from build123d import *

# Parameters (mm, degrees)
SKETCH1_R               = 51.562
SKETCH1_R_2             = 50.8
BOSS_EXTRUDE1_DEPTH     = 300
CUT_EXTRUDE1_DEPTH      = 309.73496674
CUT_EXTRUDE1_DEPTH_BACK = 309.73496674
SKETCH3_R               = 6.35
SKETCH4_R               = 3.048
SKETCH4_R_2             = 2.54
CUT_EXTRUDE2_DEPTH      = 309.734966871
CIRPATTERN1_COUNT       = 2
CIRPATTERN1_ANGLE       = 90


with BuildPart() as part:
    # Sketch1 → Boss-Extrude1 (new, symmetric)
    with BuildSketch(Plane(origin=(0, 0, 0), x_dir=(0, 0, -1), z_dir=(1, 0, 0))):
        Circle(SKETCH1_R)
        Circle(SKETCH1_R_2, mode=Mode.SUBTRACT)
    extrude(amount=BOSS_EXTRUDE1_DEPTH, both=True)

    # Sketch3 → Cut-Extrude1 (cut, two sides: drawn at the far end of the back side and taken through both)
    with BuildSketch(Plane.XY.offset(-CUT_EXTRUDE1_DEPTH_BACK)):
        with Locations((170.180000052, -8.89)):
            Circle(SKETCH3_R)
    extrude(amount=CUT_EXTRUDE1_DEPTH + CUT_EXTRUDE1_DEPTH_BACK, mode=Mode.SUBTRACT)

    # Sketch4 → Cut-Extrude2 (cut, symmetric)
    with BuildSketch(Plane.XY):
        with Locations((-287.3, 0)):
            Circle(SKETCH4_R)
        with Locations((289.586, 0)):
            Circle(SKETCH4_R_2)
    cut_extrude2 = extrude(amount=CUT_EXTRUDE2_DEPTH, both=True, mode=Mode.SUBTRACT)

    # CirPattern1: Cut-Extrude2 ×2 about axis
    cirpattern1_axis = Axis((300, 0, 0), (-1, 0, 0))
    for i in range(1, CIRPATTERN1_COUNT):
        add(cut_extrude2.rotate(cirpattern1_axis, i * CIRPATTERN1_ANGLE / (CIRPATTERN1_COUNT - 1)), mode=Mode.SUBTRACT)


solid = part.part
Work out the finished part from the listing and answer in its coordinate system (mm). Give positions to 0.01 mm unless a question says otherwise; leave off trailing zeros. Loops run counter-clockwise (first coordinate to the right, second up) from the corner with the lowest first, then second, coordinate; pieces in that order, holes last. Notation, with made-up numbers: (45.25, 62) - (80.25, 62) arc R21 cw to (80.25, 77) - close; hole circle Ø11 at (66.25, -31). An arc over 180 degrees is marked (long way). Answer in a Markdown table with one row per item. Add a question column.
Q1. The part is cut by section B-B (y = 33.5). Determine the outline of the cut face in (x, z).
Q2. Consider line 1 along X through (y, z) = (-51, 0); line 2 along Y through (x, z) = (4, 0); line 3 along Y through (x, z) = (167.5, -41). Determine where each line is inside the solid, lowest interval first.
Q3. Each of these flat-tipped pins is pushed along its axis until it touches: P1, Ø5, axis at x = 60, z = -21.5, coming from the -Y side; P2, Ø10, axis at x = -148, z = 13.5, coming from the -Y side; P3, Ø2, axis at x = 134, z = -16.5, coming from the -Y side. Where does it stop, or does it pass through?
Q4. Determine the mould class of faces 1 (the cylindrical face through (165.256, -12.9, -49.762)), 2 (the flat face through (-300, -38, -34)), 3 (the flat face through (300, -38, -34)) for opening direction X: released by +X, released by -X, zero draft, split by the parting line, or undercut.
Q5. The part is cut by section C-C (x = 245). Determine the outline of the cut face in (y, z), and give its area (3 significant figures).
Q6. The part is cut by section A-A (z = -31). Determine the outline of the cut face in (x, y).
Solution:
| question | item | result |
|---|---|---|
| 1 | outline | (-300, -39.2) - (300, -39.2) - (300, -38.19) - (-300, -38.19) - close; (-300, 38.19) - (300, 38.19) - (300, 39.2) - (-300, 39.2) - close |
| 2 | line 1 | x = -300 to -290.35, -284.25 to 287.05, 292.13 to 300 |
| 2 | line 2 | y = -51.56 to -50.8, 50.8 to 51.56 |
| 2 | line 3 | y = -31.27 to -29.99, 29.99 to 31.27 |
| 3 | P1 | stops at y = -47.93 |
| 3 | P2 | stops at y = -50.86 |
| 3 | P3 | stops at y = -49.18 |
| 4 | face 1 | undercut |
| 4 | face 2 | released by -X |
| 4 | face 3 | released by +X |
| 5 | outline | circle Ø103.12 at (0, 0); hole circle Ø101.6 at (0, 0) |
| 5 | area | 245 mm² |
| 6 | outline | (-300, -41.2) - (300, -41.2) - (300, -40.24) - (-300, -40.24) - close; (-300, 40.24) - (300, 40.24) - (300, 41.2) - (-300, 41.2) - close |
